Geometry: final body of the model. Coordinates: model frame, mm. A direction names the side the tool comes from. Round coordinates to 2 decimals unless told otherwise and drop trailing zeros. Write each loop counter-clockwise with the first axis right and the second up, starting at its lowest first coordinate (ties: lowest second). Pieces come first, ordered by that corner, then holes. Notation, with made-up numbers: (-16, 39.25) - (2, 39.25) arc R15 ccw to (2, 59.25) - close; hole circle Ø4 at (-32.75, 63.25). An arc over 180 degrees is marked (long way). Write each question's results on one line, items separated by ' | '.
from build123d import *

# Parameters (mm, degrees)
F0_R      = 12.45
F1_DEPTH  = 12
F2_R      = 14.5
F3_DEPTH  = 3
F4_R      = 9.95
F5_DEPTH  = 70
F8_DEPTH  = 12
F10_DEPTH = 20


with BuildPart() as f1:
    # F0 (on Front) → F1 (new body)
    with BuildSketch(Plane.XZ):
        Circle(F0_R)
    extrude(amount=-F1_DEPTH)

    # F2 (on Front) → F3 (join)
    with BuildSketch(Plane.XZ):
        Circle(F2_R)
    extrude(amount=F3_DEPTH)

    # F4 (on face) → F5 (join)
    with BuildSketch(Plane.XZ.offset(3)):
        Circle(F4_R)
    extrude(amount=F5_DEPTH)

    # F7 (on offset) → F8 (cut)
    with BuildSketch(Plane.XY.offset(6)):
        with BuildLine():
            Line((-3, -55), (-3, -107.7152226879))
            Line((-3, -107.7152226879), (3, -107.7152226879))
            Line((3, -107.7152226879), (3, -55))
            ThreePointArc((3, -55), (0, -52), (-3, -55))
        make_face()
    extrude(amount=F8_DEPTH, mode=Mode.SUBTRACT)

    # F9 (on face) → F10 (join)
    with BuildSketch(Plane.XZ.offset(3)):
        with BuildLine():
            Line((-8.8706942802, 8.8068599959), (-7.3471313431, 6.7098555146))
            ThreePointArc((-7.3471313431, 6.7098555146), (-5.8484632603, 8.049719094), (-4.1110633656, 9.0609965238))
            Line((-4.1110633656, 9.0609965238), (-5.6346263027, 11.1580010051))
            ThreePointArc((-5.6346263027, 11.1580010051), (-7.3473156537, 10.1127124297), (-8.8706942802, 8.8068599959))
        make_face()
        with BuildLine():
            Line((-2, 12.3389626793), (-2, 9.7469225913))
            ThreePointArc((-2, 9.7469225913), (0, 9.95), (2, 9.7469225913))
            Line((2, 9.7469225913), (2, 12.3389626793))
            ThreePointArc((2, 12.3389626793), (0, 12.5), (-2, 12.3389626793))
        make_face()
        with BuildLine():
            ThreePointArc((4.1110633656, 9.0609965238), (5.8484632603, 8.049719094), (7.3471313431, 6.7098555146))
            Line((7.3471313431, 6.7098555146), (8.8706942802, 8.8068599959))
            ThreePointArc((8.8706942802, 8.8068599959), (7.3473156537, 10.1127124297), (5.6346263027, 11.1580010051))
            Line((5.6346263027, 11.1580010051), (4.1110633656, 9.0609965238))
        make_face()
        with BuildLine():
            ThreePointArc((8.6518402555, 4.9140777561), (9.4630123371, 3.074719094), (9.887908233, 1.109851691))
            Line((9.887908233, 1.109851691), (12.3530848492, 1.9108361283))
            ThreePointArc((12.3530848492, 1.9108361283), (11.8882064537, 3.8627124297), (11.1170168717, 5.7150621934))
            Line((11.1170168717, 5.7150621934), (8.6518402555, 4.9140777561))
        make_face()
        with BuildLine():
            ThreePointArc((9.887908233, -1.109851691), (9.4630123371, -3.074719094), (8.6518402555, -4.9140777561))
            Line((8.6518402555, -4.9140777561), (11.1170168717, -5.7150621934))
            ThreePointArc((11.1170168717, -5.7150621934), (11.8882064537, -3.8627124297), (12.3530848492, -1.9108361283))
            Line((12.3530848492, -1.9108361283), (9.887908233, -1.109851691))
        make_face()
        with BuildLine():
            Line((-12.3530848492, 1.9108361283), (-9.887908233, 1.109851691))
            ThreePointArc((-9.887908233, 1.109851691), (-9.4630123371, 3.074719094), (-8.6518402555, 4.9140777561))
            Line((-8.6518402555, 4.9140777561), (-11.1170168717, 5.7150621934))
            ThreePointArc((-11.1170168717, 5.7150621934), (-11.8882064537, 3.8627124297), (-12.3530848492, 1.9108361283))
        make_face()
        with BuildLine():
            Line((-11.1170168717, -5.7150621934), (-8.6518402555, -4.9140777561))
            ThreePointArc((-8.6518402555, -4.9140777561), (-9.4630123371, -3.074719094), (-9.887908233, -1.109851691))
            Line((-9.887908233, -1.109851691), (-12.3530848492, -1.9108361283))
            ThreePointArc((-12.3530848492, -1.9108361283), (-11.8882064537, -3.8627124297), (-11.1170168717, -5.7150621934))
        make_face()
        with BuildLine():
            Line((-5.6346263027, -11.1580010051), (-4.1110633656, -9.0609965238))
            ThreePointArc((-4.1110633656, -9.0609965238), (-5.8484632603, -8.049719094), (-7.3471313431, -6.7098555146))
            Line((-7.3471313431, -6.7098555146), (-8.8706942802, -8.8068599959))
            ThreePointArc((-8.8706942802, -8.8068599959), (-7.3473156537, -10.1127124297), (-5.6346263027, -11.1580010051))
        make_face()
        with BuildLine():
            Line((-2, -9.7469225913), (-2, -12.3389626793))
            ThreePointArc((-2, -12.3389626793), (0, -12.5), (2, -12.3389626793))
            Line((2, -12.3389626793), (2, -9.7469225913))
            ThreePointArc((2, -9.7469225913), (0, -9.95), (-2, -9.7469225913))
        make_face()
        with BuildLine():
            ThreePointArc((7.3471313431, -6.7098555146), (5.8484632603, -8.049719094), (4.1110633656, -9.0609965238))
            Line((4.1110633656, -9.0609965238), (5.6346263027, -11.1580010051))
            ThreePointArc((5.6346263027, -11.1580010051), (7.3473156537, -10.1127124297), (8.8706942802, -8.8068599959))
            Line((8.8706942802, -8.8068599959), (7.3471313431, -6.7098555146))
        make_face()
    extrude(amount=F10_DEPTH)


solid = f1.part
Q1. Access query for faces 1 (the flat face through (2, -13, 11)), 2 (the cylindrical face through (-11.897, -12.86, -3.836)), 3 (the flat face through (-11.103, -12.86, -1.505)), 4 (the cylindrical face through (7.37, -12.86, 10.096)). Directions: +Z, -Z, +X, -X, +Y, -Y. A direction counts if a zero-diameter tool reaches every point of the face in a straight line with its end or side. Return the directions, or none.
Answer block:
face 1: +Z, -Y | face 2: -Z, -X, -Y | face 3: -X, -Y | face 4: +Z, +X, -Y
Q2. Section query D-D, the plane x = -6.5. Return loops of the section in (y, z).
Answer block:
outline: (-73, -7.53) - (-23, -7.53) - (-23, -10.68) - (-3, -10.68) - (-3, -12.96) - (0, -12.96) - (0, -10.62) - (12, -10.62) - (12, 10.62) - (0, 10.62) - (0, 12.96) - (-3, 12.96) - (-3, 10.68) - (-23, 10.68) - (-23, 7.53) - (-73, 7.53) - close
Q3. Pin query (flat end, axial travel): pin 1 (3.5 mm diameter, centred on x = 7, z = 9.5, fed in from -Y); pin 2 (8 mm diameter, centred on x = 5.5, y = -31, fed in from -Z); pin 3 (1 mm diameter, centred on y = -67, z = 7.5, fed in from -X). Return the tip coordinate at first contact, or that it passes through.
Answer block:
pin 1: y = -23 | pin 2: z = -9.84 | pin 3: x = -7.07
Q4. Mould query, pull axis X, two halves, no side actions, for faces 5 (the flat face through (6, -23, 9)), 6 (the flat face through (-8.098, -12.86, -7.744)), 7 (the flat face through (4.86, -12.86, -10.09)). Classes: pulls with the +X half, pulls with the -X half, needs draft (parallel to the pull), parting line crosses it, or undercut.
Answer block:
face 5: needs draft | face 6: pulls with the -X half | face 7: undercut
Q5. Section query C-C, the plane y = -48. Return loops of the section in (x, z).
Answer block:
outline: circle Ø19.9 at (0, 0)
Q6. Section query B-B, the plane z = 0. Return loops of the section in (x, y).
Answer block:
outline: (-14.5, -3) - (-9.95, -3) - (-9.95, -73) - (9.95, -73) - (9.95, -3) - (14.5, -3) - (14.5, 0) - (12.45, 0) - (12.45, 12) - (-12.45, 12) - (-12.45, 0) - (-14.5, 0) - close
Q7. Ray query, line 1 along Z through (x, y) = (-7.75, -4.5); line 2 along Z through (x, y) = (1.5, 3.5); line 3 along Y through (x, z) = (2.75, -13). Return the intervals inside material, ascending.
Answer block:
line 1: -9.81 to -7.26, -6.24 to 6.24, 7.26 to 9.81 | line 2: -12.36 to 12.36 | line 3: -3 to 0
Q8. Section query A-A, the plane x = 0. Return loops of the section in (y, z), plus the area to 3 significant figures.
Answer block:
outline: (-73, -9.95) - (-23, -9.95) - (-23, -12.5) - (-3, -12.5) - (-3, -14.5) - (0, -14.5) - (0, -12.45) - (12, -12.45) - (12, 12.45) - (0, 12.45) - (0, 14.5) - (-3, 14.5) - (-3, 12.5) - (-23, 12.5) - (-23, 9.95) - (-52, 9.95) - (-52, 6) - (-73, 6) - close | area: 1,800 mm2
